```python
from build123d import *

# Parameters (mm, degrees)
SZKIC1_R                    = 3.5
DODANIE_WYCI_GNI_CIE1_DEPTH = 9
SZKIC2_R                    = 1.9
WYTNIJ_WYCI_GNI_CIE1_DEPTH  = 3.5
SZKIC3_R                    = 2
DODANIE_WYCI_GNI_CIE2_DEPTH = 1.6
WYTNIJ_WYCI_GNI_CIE2_START  = -0.6
SZKIC4_R                    = 2.15
WYTNIJ_WYCI_GNI_CIE2_DEPTH  = 0.6
SZKIC5_R                    = 1
WYTNIJ_WYCI_GNI_CIE3_DEPTH  = 31.6
SZKIC6_R                    = 3.5
SZKIC6_R_2                  = 2.75
WYTNIJ_WYCI_GNI_CIE4_DEPTH  = 0.6


with BuildPart() as part:
    # Szkic1 → Dodanie-wyciągnięcie1 (new body)
    with BuildSketch(Plane(origin=(0, 0, 0), x_dir=(1, 0, 0), z_dir=(0, 1, 0))):
        Circle(SZKIC1_R)
    extrude(amount=DODANIE_WYCI_GNI_CIE1_DEPTH)

    # Szkic2 → Wytnij-wyciągnięcie1 (cut)
    with BuildSketch(Plane.XZ):
        Circle(SZKIC2_R)
    extrude(amount=-WYTNIJ_WYCI_GNI_CIE1_DEPTH, mode=Mode.SUBTRACT)

    # Szkic3 → Dodanie-wyciągnięcie2 (add)
    with BuildSketch(Plane(origin=(0, 8.4, 0), x_dir=(1, 0, 0), z_dir=(0, 1, 0))):
        with Locations((-8.95, 0)):
            Circle(SZKIC3_R)
        with BuildLine():
            Line((-2, 2), (-8.95, 2))
            ThreePointArc((-8.95, 2), (-7.535786438, 1.414213562), (-6.95, 0))
            ThreePointArc((-6.95, 0), (-7.535786438, -1.414213562), (-8.95, -2))
            Line((-8.95, -2), (-2, -2))
            Line((-2, -2), (-2, 2))
        make_face()
        with Locations((0, 7)):
            Circle(SZKIC3_R)
        with BuildLine():
            Line((-2, 7), (-2, 2))
            Line((-2, 2), (0, 2))
            Line((0, 2), (2, 2))
            Line((2, 2), (2, 7))
            ThreePointArc((2, 7), (0, 5), (-2, 7))
        make_face()
        with BuildLine():
            Line((8.95, 2), (2, 2))
            Line((2, 2), (2, 0))
            Line((2, 0), (2, -2))
            Line((2, -2), (8.95, -2))
            ThreePointArc((8.95, -2), (6.95, 0), (8.95, 2))
        make_face()
        with Locations((8.95, 0)):
            Circle(SZKIC3_R)
        with Locations((0, -7)):
            Circle(SZKIC3_R)
        with BuildLine():
            Line((2, -2), (-2, -2))
            Line((-2, -2), (-2, -7))
            ThreePointArc((-2, -7), (0, -5), (2, -7))
            Line((2, -7), (2, -2))
        make_face()
    extrude(amount=-DODANIE_WYCI_GNI_CIE2_DEPTH)

    # Szkic4 → Wytnij-wyciągnięcie2 (cut)
    with BuildSketch(Plane(origin=(0, 9, 0), x_dir=(1, 0, 0), z_dir=(0, 1, 0)).offset(WYTNIJ_WYCI_GNI_CIE2_START)):
        Circle(SZKIC4_R)
    extrude(amount=WYTNIJ_WYCI_GNI_CIE2_DEPTH, mode=Mode.SUBTRACT)

    # Szkic5 → Wytnij-wyciągnięcie3 (cut)
    with BuildSketch(Plane(origin=(0, 8.4, 0), x_dir=(1, 0, 0), z_dir=(0, 1, 0))):
        Circle(SZKIC5_R)
    extrude(amount=-WYTNIJ_WYCI_GNI_CIE3_DEPTH, mode=Mode.SUBTRACT)

    # Szkic6 → Wytnij-wyciągnięcie4 (cut)
    with BuildSketch(Plane(origin=(0, 9, 0), x_dir=(1, 0, 0), z_dir=(0, 1, 0))):
        Circle(SZKIC6_R)
        Circle(SZKIC6_R_2, mode=Mode.SUBTRACT)
    extrude(amount=-WYTNIJ_WYCI_GNI_CIE4_DEPTH, mode=Mode.SUBTRACT)


solid = part.part
```
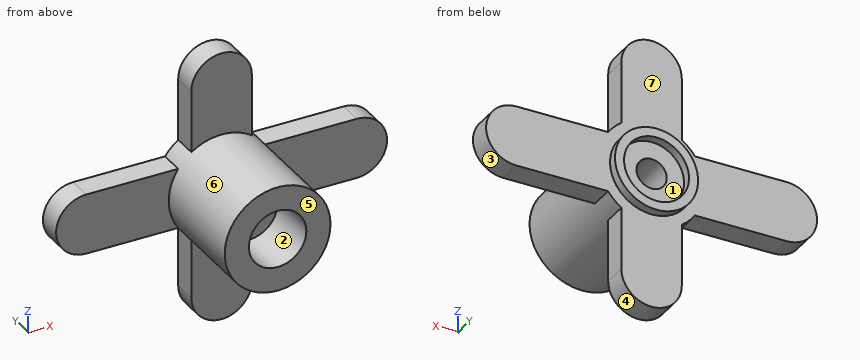
CAD build for the part. Positions are in the model's coordinates, mm. Face numbers are marked on the shaded views. A direction names the side the tool comes from. Give positions to 0.01 mm unless a question says otherwise; leave off trailing zeros. Loops run counter-clockwise (first coordinate to the right, second up) from the corner with the lowest first, then second, coordinate; pieces in that order, holes last. Notation, with made-up numbers: (34.5, 30) -> (40.5, 30) arc R23 ccw to (40.5, 44) -> close; hole circle Ø5 at (39.25, 14). An arc over 180 degrees is marked (long way). Use a Markdown table: item, result.
1. Slice it at C-C (x = 3.25). List the corners of the cut face in (y, z).
Check result:
| item | result |
|---|---|
| outline | (0, -1.3) -> (6.8, -1.3) -> (6.8, -2) -> (8.4, -2) -> (8.4, 2) -> (6.8, 2) -> (6.8, 1.3) -> (0, 1.3) -> close |
2. Wall check: L1, parallel to X at y = 8.7, z = 0; L2, parallel to X at y = 6.65, z = 0; L3, parallel to Z at x = 0, y = 1.2. Give the ranges that are in metal, low to high. Write a range as [from, to].
Check result:
| item | result |
|---|---|
| L1 | x = [-2.75, -2.15], [2.15, 2.75] |
| L2 | x = [-3.5, -1], [1, 3.5] |
| L3 | z = [-3.5, -1.9], [1.9, 3.5] |
3. Slice it at D-D (z = -4). List the corners of the cut face in (x, y), plus the area to 3 significant figures.
Check result:
| item | result |
|---|---|
| outline | (-2, 6.8) -> (2, 6.8) -> (2, 8.4) -> (-2, 8.4) -> close |
| area | 6.40 mm^2 |
4. Slice it at A-A (x = 0). List the corners of the cut face in (y, z).
Check result:
| item | result |
|---|---|
| outline | (0, -3.5) -> (6.8, -3.5) -> (6.8, -9) -> (8.4, -9) -> (8.4, -2.75) -> (9, -2.75) -> (9, -2.15) -> (8.4, -2.15) -> (8.4, -1) -> (3.5, -1) -> (3.5, -1.9) -> (0, -1.9) -> close; (0, 1.9) -> (3.5, 1.9) -> (3.5, 1) -> (8.4, 1) -> (8.4, 2.15) -> (9, 2.15) -> (9, 2.75) -> (8.4, 2.75) -> (8.4, 9) -> (6.8, 9) -> (6.8, 3.5) -> (0, 3.5) -> close |
5. Slice it at B-B (y = 3). List the corners of the cut face in (x, z), plus the area to 3 significant figures.
Check result:
| item | result |
|---|---|
| outline | circle Ø7 at (0, 0); hole circle Ø3.8 at (0, 0) |
| area | 27.1 mm^2 |
6. Which spindle directions (+Z, -Z, +X, -X, +Y, -Y) get a long thin tool onto all of the face, cutting with end or side? Do the marked faces 5, 6 and 7. Say none if no direction does.
Check result:
| item | result |
|---|---|
| face 5 | +Z, -Z, +X, -X, -Y |
| face 6 | -Y |
| face 7 | +Y |
7. Mould opens along Z. For the marked faces 1, 2, 3 and 4 say: pulls with the +Z half, pulls with the -Z half, needs draft (parallel to the pull), parting line crosses it, or undercut.
Check result:
| item | result |
|---|---|
| face 1 | undercut |
| face 2 | undercut |
| face 3 | parting line crosses it |
| face 4 | pulls with the -Z half |
8. Flat gauge pins, fed straight in: pin 1 (3 mm diameter, centred on x = 0, z = 0, fed in from -Y); pin 2 (1.3 mm diameter, centred on y = 7.5, z = -5, fed in from +X); pin 3 (1.8 mm diameter, centred on x = 5, y = 7.5, fed in from -Z). Where does each tip first touch, or does it go through?
Check result:
| item | result |
|---|---|
| pin 1 | stops at y = 3.5 |
| pin 2 | stops at x = 2 |
| pin 3 | stops at z = -2 |
